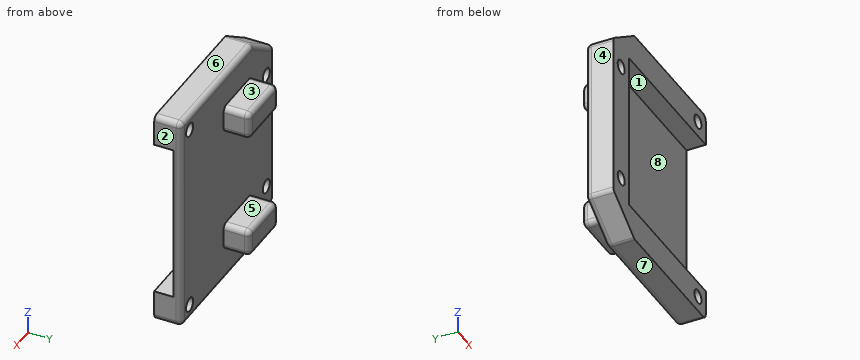
from build123d import *

# Parameters (mm, degrees)
SKETCH1_W           = 32.9
SKETCH1_H           = 40.2
BOSS_EXTRUDE1_DEPTH = 5
SKETCH2_W           = 29
SKETCH2_H           = 3.5
CUT_EXTRUDE1_DEPTH  = 27.3
SKETCH3_R           = 1.25
CUT_EXTRUDE2_DEPTH  = 6
SKETCH4_W           = 10
SKETCH4_H           = 5
BOSS_EXTRUDE2_DEPTH = 4.7625
CHAMFER1_SIZE       = 7.5
CHAMFER1_SIZE2      = 5.1
CHAMFER2_SIZE       = 5.1
CHAMFER2_SIZE2      = 7.5
FILLET1_R           = 1


with BuildPart() as part:
    # Sketch1 → Boss-Extrude1 (new body)
    with BuildSketch(Plane(origin=(0, 0, 0), x_dir=(1, 0, 0), z_dir=(0, 1, 0))):
        Rectangle(SKETCH1_W, SKETCH1_H)
    extrude(amount=BOSS_EXTRUDE1_DEPTH)

    # Sketch2 → Cut-Extrude1 (cut)
    with BuildSketch(Plane(origin=(16.45, 0, 0), x_dir=(0, 0, -1), z_dir=(1, 0, 0))):
        with Locations((0, 1.75)):
            Rectangle(SKETCH2_W, SKETCH2_H)
    extrude(amount=-CUT_EXTRUDE1_DEPTH, mode=Mode.SUBTRACT)

    # Sketch3 → Cut-Extrude2 (cut, through all)
    with BuildSketch(Plane(origin=(0, 5, 0), x_dir=(1, 0, 0), z_dir=(0, 1, 0))):
        with Locations((13.65, 17.3)):
            Circle(SKETCH3_R)
        with Locations((-13.65, 11)):
            Circle(SKETCH3_R)
    cut_extrude2 = extrude(amount=-CUT_EXTRUDE2_DEPTH, mode=Mode.SUBTRACT)

    # Sketch4 → Boss-Extrude2 (add)
    with BuildSketch(Plane(origin=(0, 5, 0), x_dir=(-1, 0, 0), z_dir=(0, 1, 0))):
        with Locations((3.45, -11.6)):
            Rectangle(SKETCH4_W, SKETCH4_H)
    boss_extrude2 = extrude(amount=BOSS_EXTRUDE2_DEPTH)

    # Mirror1: Cut-Extrude2, Boss-Extrude2 across plane
    add(cut_extrude2.mirror(Plane.XY), mode=Mode.SUBTRACT)
    add(boss_extrude2.mirror(Plane.XY))

    # Chamfer1
    chamfer1_edges = [part.edges().sort_by_distance(p)[0] for p in [
        (-16.45, 2.5, -20.1),
    ]]
    chamfer1_side = [part.faces().sort_by_distance(p)[0] for p in [
        (0, 2.5, -20.1),
    ]]
    chamfer(chamfer1_edges, length=CHAMFER1_SIZE, length2=CHAMFER1_SIZE2, reference=chamfer1_side[0])

    # Chamfer2
    chamfer2_edges = [part.edges().sort_by_distance(p)[0] for p in [
        (-16.45, 2.5, 20.1),
    ]]
    chamfer2_side = [part.faces().sort_by_distance(p)[0] for p in [
        (-16.45, 2.5, 2.55),
    ]]
    chamfer(chamfer2_edges, length=CHAMFER2_SIZE, length2=CHAMFER2_SIZE2, reference=chamfer2_side[0])

    # Fillet1
    fillet1_edges = [part.edges().sort_by_distance(p)[0] for p in [
        (1.55, 7.38125, -9.1),
        (1.55, 7.38125, -14.1),
        (16.45, 5, 0),
        (-8.45, 7.38125, -14.1),
        (-8.45, 7.38125, -9.1),
        (1.55, 9.7625, -11.6),
        (-3.45, 9.7625, -14.1),
        (-8.45, 9.7625, -11.6),
        (-3.45, 9.7625, -9.1),
        (1.55, 9.7625, 11.6),
        (1.55, 7.38125, 14.1),
        (-3.45, 9.7625, 9.1),
        (1.55, 7.38125, 9.1),
        (-8.45, 9.7625, 11.6),
        (-8.45, 7.38125, 9.1),
        (-3.45, 9.7625, 14.1),
        (-8.45, 7.38125, 14.1),
        (3.75, 5, -20.1),
        (-16.45, 5, 0),
        (-16.45, 2.5, -15),
        (-8.95, 2.5, -20.1),
        (-12.7, 5, -17.55),
        (16.45, 2.5, 20.1),
        (3.75, 5, 20.1),
        (-8.95, 2.5, 20.1),
        (16.45, 2.5, -20.1),
        (-16.45, 2.5, 15),
        (-12.7, 5, 17.55),
    ]]
    fillet(fillet1_edges, radius=FILLET1_R)


solid = part.part
Check sheet for the modelled part. Datum: model origin and axes. Units: mm. Face numbers are marked on the shaded views. A direction names the side the tool comes from. Coordinates: 2 decimals unless noted, no trailing zeros. Write each loop counter-clockwise with the first axis right and the second up, starting at its lowest first coordinate (ties: lowest second). Pieces come first, ordered by that corner, then holes.
Item 1: Depth check by flat-ended pin: pin 1 Ø1.5 at (y, z) = (1, -12) entering from +X; pin 2 Ø12 at (x, z) = (4, 1.5) entering from -Y; pin 3 Ø8 at (x, z) = (3.5, 0.5) entering from +Y. Enter the tip coordinate at first touch or a pass-through.
Numbers:
pin 1: stops at x = -10.85
pin 2: stops at y = 3.5
pin 3: stops at y = 5
Item 2: Cross-section at B-B on z = -11. Record the boundary of the cut face in (x, y).
Numbers:
outline: (-16.45, 0) - (-14.9, 0) - (-14.9, 5) - (-15.45, 5) arc R1 ccw to (-16.45, 4) - close; (-12.4, 0) - (-10.85, 0) - (-10.85, 3.5) - (16.45, 3.5) - (16.45, 4) arc R1 ccw to (15.45, 5) - (1.55, 5) - (1.55, 8.76) arc R1 ccw to (0.55, 9.76) - (-7.45, 9.76) arc R1 ccw to (-8.45, 8.76) - (-8.45, 5) - (-12.4, 5) - close
Item 3: Scan lines: probe 1 along Z at (x, y) = (13.65, 2.6); probe 2 along Z at (x, y) = (2.5, 1); probe 3 along X at (y, z) = (2.7, 11). Record each from-to range of solid material in increasing order.
Numbers:
probe 1: z = -20.1 to -18.55, -16.05 to -14.5, 14.5 to 16.05, 18.55 to 20.1
probe 2: z = -20.1 to -14.5, 14.5 to 20.1
probe 3: x = -16.45 to -14.9, -12.4 to -10.85
Item 4: Mould release check, pull along Z, two halves, no side actions. Record for the marked faces 6, 7 and 8: released by +Z, released by -Z, zero draft, split by the parting line, or undercut.
Numbers:
face 6: released by +Z
face 7: released by -Z
face 8: undercut
Item 5: Cross-section at C-C on z = 6.5. Record the boundary of the cut face in (x, y), then the cut area to 3 significant figures.
Numbers:
outline: (-16.45, 0) - (-10.85, 0) - (-10.85, 3.5) - (16.45, 3.5) - (16.45, 4) arc R1 ccw to (15.45, 5) - (-15.45, 5) arc R1 ccw to (-16.45, 4) - close
area: 68.5 mm2
Item 6: Cross-section at A-A on x = 13.65. Record the boundary of the cut face in (y, z).
Numbers:
outline: (0, -20.1) - (4, -20.1) arc R1 ccw to (5, -19.1) - (5, -18.55) - (0, -18.55) - close; (0, -16.05) - (5, -16.05) - (5, 16.05) - (0, 16.05) - (0, 14.5) - (3.5, 14.5) - (3.5, -14.5) - (0, -14.5) - close; (0, 18.55) - (5, 18.55) - (5, 19.1) arc R1 ccw to (4, 20.1) - (0, 20.1) - close
Item 7: Access from +Z, -Z, +X, -X, +Y, -Y to the whole of each face (thin tool, end or side, straight path). Record for the marked faces 1, 2, 3, 4 and 5.
Numbers:
face 1: +X, -Y
face 2: +Z, -Z, +X, +Y, -Y
face 3: +Z, +X, -X, +Y
face 4: +Z, -Z, -X, +Y, -Y
face 5: +X, -X, +Y
Item 8: Cross-section at D-D on x = -2. Record the boundary of the cut face in (y, z).
Numbers:
outline: (0, -20.1) - (4, -20.1) arc R1 ccw to (5, -19.1) - (5, -14.1) - (8.76, -14.1) arc R1 ccw to (9.76, -13.1) - (9.76, -10.1) arc R1 ccw to (8.76, -9.1) - (5, -9.1) - (5, 9.1) - (8.76, 9.1) arc R1 ccw to (9.76, 10.1) - (9.76, 13.1) arc R1 ccw to (8.76, 14.1) - (5, 14.1) - (5, 19.1) arc R1 ccw to (4, 20.1) - (0, 20.1) - (0, 14.5) - (3.5, 14.5) - (3.5, -14.5) - (0, -14.5) - close
